Here's how the part is built. I have some questions about the finished solid (model axes, mm). A direction names the side the tool comes from. Round coordinates to 2 decimals unless told otherwise and drop trailing zeros. Write each loop counter-clockwise with the first axis right and the second up, starting at its lowest first coordinate (ties: lowest second). Pieces come first, ordered by that corner, then holes. Notation, with made-up numbers: (81.25, 74) -> (108.25, 74) arc R27 ccw to (108.25, 103) -> close; hole circle Ø5 at (73, 40.5). An arc over 180 degrees is marked (long way). Answer as CSV lines item,"result".
from build123d import *

# Parameters (mm, degrees)
BOSS_EXTRUDE1_DEPTH = 10.75
SKETCH2_R           = 3
SKETCH2_R_2         = 5
BOSS_EXTRUDE2_DEPTH = 2
SKETCH3_R           = 1.5
CUT_EXTRUDE1_DEPTH  = 6
SKETCH4_R           = 3
BOSS_EXTRUDE3_DEPTH = 13.7
SKETCH5_R           = 12.2
BOSS_EXTRUDE4_DEPTH = 31


with BuildPart() as part:
    # Sketch1 → Boss-Extrude1 (new, symmetric)
    with BuildSketch(Plane(origin=(0, 0, 0), x_dir=(1, 0, 0), z_dir=(0, 1, 0))):
        with BuildLine():
            Line((-20.5, -16), (20.5, -16))
            ThreePointArc((20.5, -16), (22.267766953, -15.267766953), (23, -13.5))
            Line((23, -13.5), (23, 13.5))
            ThreePointArc((23, 13.5), (22.267766953, 15.267766953), (20.5, 16))
            Line((20.5, 16), (-20.5, 16))
            ThreePointArc((-20.5, 16), (-22.267766953, 15.267766953), (-23, 13.5))
            Line((-23, 13.5), (-23, -13.5))
            ThreePointArc((-23, -13.5), (-22.267766953, -15.267766953), (-20.5, -16))
        make_face()
    extrude(amount=BOSS_EXTRUDE1_DEPTH, both=True)

    # Sketch2 → Boss-Extrude2 (add)
    with BuildSketch(Plane(origin=(0, 10.75, 0), x_dir=(1, 0, 0), z_dir=(0, 1, 0))):
        with Locations(Location((-16.5, 9, 0), (0, 0, 270))):
            Circle(SKETCH2_R)
        with Locations(Location((-16.5, -9, 0), (0, 0, 270))):
            Circle(SKETCH2_R)
        with Locations(Location((16.5, -9, 0), (0, 0, 270))):
            Circle(SKETCH2_R)
        with Locations(Location((16.5, 9, 0), (0, 0, 270))):
            Circle(SKETCH2_R)
        with Locations(Location((-7.5, 0, 0), (0, 0, 270))):
            Circle(SKETCH2_R_2)
    extrude(amount=BOSS_EXTRUDE2_DEPTH)

    # Sketch3 → Cut-Extrude1 (cut)
    with BuildSketch(Plane(origin=(0, 12.75, 0), x_dir=(1, 0, 0), z_dir=(0, 1, 0))):
        with Locations(Location((-16.5, 9, 0), (0, 0, 270))):
            Circle(SKETCH3_R)
        with Locations(Location((16.5, 9, 0), (0, 0, 270))):
            Circle(SKETCH3_R)
        with Locations(Location((16.5, -9, 0), (0, 0, 270))):
            Circle(SKETCH3_R)
        with Locations(Location((-16.5, -9, 0), (0, 0, 270))):
            Circle(SKETCH3_R)
    extrude(amount=-CUT_EXTRUDE1_DEPTH, mode=Mode.SUBTRACT)

    # Sketch4 → Boss-Extrude3 (add)
    with BuildSketch(Plane(origin=(0, 12.75, 0), x_dir=(1, 0, 0), z_dir=(0, 1, 0))):
        with Locations(Location((-7.5, 0, 0), (0, 0, 90))):
            Circle(SKETCH4_R)
    extrude(amount=BOSS_EXTRUDE3_DEPTH)

    # Sketch5 → Boss-Extrude4 (add)
    with BuildSketch(Plane(origin=(23, 0, 0), x_dir=(0, 0, -1), z_dir=(1, 0, 0))):
        with Locations(Location((2.436698586, -1.75, 0), (0, 0, 227.536275048))):
            Circle(SKETCH5_R)
    extrude(amount=BOSS_EXTRUDE4_DEPTH)


solid = part.part
Item 1: Suppose I cut it at A-A, the plane y = -1.75. List the corners of the cut face in (x, z) for me.
Results found:
outline,"(-23, -13.5) arc R2.5 ccw to (-20.5, -16) -> (20.5, -16) arc R2.5 ccw to (23, -13.5) -> (23, -14.64) -> (54, -14.64) -> (54, 9.76) -> (23, 9.76) -> (23, 13.5) arc R2.5 ccw to (20.5, 16) -> (-20.5, 16) arc R2.5 ccw to (-23, 13.5) -> close"
Item 2: If we mould it in two halves opening along Z, with no side actions, what happens to faces 4 (the flat face through (-15, 12.75, -8)), 5 (the cylindrical face through (38.28, -0.68, -14.59)), 6 (the flat face through (17, 6.75, -9))? For each: pulls with the +Z half, pulls with the -Z half, needs draft (parallel to the pull), parting line crosses it, or undercut.
Results found:
face 4,"needs draft"
face 5,"parting line crosses it"
face 6,"undercut"
Item 3: Suppose I cut it at B-B, the plane x = -7.5. List the corners of the cut face in (y, z) for me.
Results found:
outline,"(-10.75, -16) -> (10.75, -16) -> (10.75, -5) -> (12.75, -5) -> (12.75, -3) -> (26.45, -3) -> (26.45, 3) -> (12.75, 3) -> (12.75, 5) -> (10.75, 5) -> (10.75, 16) -> (-10.75, 16) -> close"
Item 4: Will these pins go through, and if not, where does the flat tip stop? pin 1 (0.9 mm diameter, centred on x = 16.5, z = -9.5, fed in from +Y); pin 2 (12 mm diameter, centred on x = 23.5, z = 7.5, fed in from +Y); pin 3 (5 mm diameter, centred on x = -12.5, z = 3.5, fed in from -Y); pin 4 (1.5 mm diameter, centred on x = 34, z = 11, fed in from +Y).
Results found:
pin 1,"stops at y = 6.75"
pin 2,"stops at y = 12.75"
pin 3,"stops at y = -10.75"
pin 4,"passes through"
Item 5: For faces 1 (the flat face through (18, 12.75, 10)), 2 (the flat face through (-10, 12.75, 2)), 3 (the flat face through (0, -10.75, 0)), which set-ups out of +Z, -Z, +X, -X, +Y, -Y let a thin tool reach every point of the face, with its end or its side?
Results found:
face 1,"+Z, -Z, +X, -X, +Y"
face 2,"+Y"
face 3,"+Z, -Z, -X, -Y"
Item 6: Suppose I cut it at C-C, the plane z = 9. List the corners of the cut face in (x, y) for me.
Results found:
outline,"(-23, -10.75) -> (23, -10.75) -> (23, -6) -> (54, -6) -> (54, 2.5) -> (23, 2.5) -> (23, 10.75) -> (19.5, 10.75) -> (19.5, 12.75) -> (18, 12.75) -> (18, 6.75) -> (15, 6.75) -> (15, 12.75) -> (13.5, 12.75) -> (13.5, 10.75) -> (-13.5, 10.75) -> (-13.5, 12.75) -> (-15, 12.75) -> (-15, 6.75) -> (-18, 6.75) -> (-18, 12.75) -> (-19.5, 12.75) -> (-19.5, 10.75) -> (-23, 10.75) -> close"
Item 7: I need wall thicknesses on L1, parallel to X at y = 11.45, z = 9; L2, parallel to X at y = 9.7, z = 9; L3, parallel to Y at x = -15, z = -2.5. Which ranges of each line are inside material? Lowest first, please.
Results found:
L1,"x = -19.5 to -18, -15 to -13.5, 13.5 to 15, 18 to 19.5"
L2,"x = -23 to -18, -15 to 15, 18 to 23"
L3,"y = -10.75 to 10.75"
Item 8: Suppose I cut it at D-D, the plane x = -16.5. List the corners of the cut face in (y, z) for me, then the cut area to 3 significant figures.
Results found:
outline,"(-10.75, -16) -> (10.75, -16) -> (10.75, -12) -> (12.75, -12) -> (12.75, -10.5) -> (6.75, -10.5) -> (6.75, -7.5) -> (12.75, -7.5) -> (12.75, -6) -> (10.75, -6) -> (10.75, 6) -> (12.75, 6) -> (12.75, 7.5) -> (6.75, 7.5) -> (6.75, 10.5) -> (12.75, 10.5) -> (12.75, 12) -> (10.75, 12) -> (10.75, 16) -> (-10.75, 16) -> close"
area,"676 mm²"
